Could you check a few things on this model? Use its own coordinates, in mm. A direction names the side the tool comes from. Round coordinates to 2 decimals unless told otherwise and drop trailing zeros. Loops run counter-clockwise (first coordinate to the right, second up) from the corner with the lowest first, then second, coordinate; pieces in that order, holes last.
from build123d import *

# Parameters (mm, degrees)
BASE_FLANGE1_DEPTH        = 3.175
EDGE_FLANGE1_DEPTH        = 95.421779032
EDGE_FLANGE1_BEND_DEPTH   = 168.275
EDGE_FLANGE1_BEND_2_DEPTH = 76.2


# Sheet-metal steps are written as plain solids
with BuildPart() as part:
    # Sketch1 → Base-Flange1 (new body)
    with BuildSketch(Plane(origin=(0, 0, 0), x_dir=(1, 0, 0), z_dir=(0, 1, 0))):
        Polygon((168.275, 79.375), (72.853220968, 79.375), (0, 28.362625496), (0, 6.35), (168.275, 6.35), align=None)
    extrude(amount=-BASE_FLANGE1_DEPTH)

    # Edge-Flange1 section (across the edge) → Edge-Flange1 (add)
    with BuildSketch(Plane(origin=(168.275, 0, -82.55), x_dir=(0, 0, 1), z_dir=(-1, 0, 0))):
        with BuildLine():
            Line((-3.175, 3.175), (-3.175, 15.875))
            Line((-3.175, 15.875), (0, 15.875))
            Line((0, 15.875), (0, 3.175))
            ThreePointArc((0, 3.175), (0.92993597, 0.92993597), (3.175, 0))
            Line((3.175, 0), (3.175, -3.175))
            ThreePointArc((3.175, -3.175), (-1.315128061, -1.315128061), (-3.175, 3.175))
        make_face()
    extrude(amount=EDGE_FLANGE1_DEPTH)

    # Edge-Flange1 section 2 (across the edge) → Edge-Flange1 bend (add)
    with BuildSketch(Plane(origin=(0, 0, -3.175), x_dir=(0, 0, -1), z_dir=(1, 0, 0))):
        with BuildLine():
            Line((-3.175, 3.175), (-3.175, 15.875))
            Line((-3.175, 15.875), (0, 15.875))
            Line((0, 15.875), (0, 3.175))
            ThreePointArc((0, 3.175), (0.92993597, 0.92993597), (3.175, 0))
            Line((3.175, 0), (3.175, -3.175))
            ThreePointArc((3.175, -3.175), (-1.315128061, -1.315128061), (-3.175, 3.175))
        make_face()
    extrude(amount=EDGE_FLANGE1_BEND_DEPTH)

    # Edge-Flange1 section 3 (across the edge) → Edge-Flange1 bend 2 (add)
    with BuildSketch(Plane(origin=(60.598280589, 0, -74.669957686), x_dir=(0.5735764363510473, 3.491481338843133e-15, 0.819152044288991), z_dir=(-0.819152044288991, 0, 0.5735764363510473))):
        with BuildLine():
            Line((-3.175, 3.175), (-3.175, 15.875))
            Line((-3.175, 15.875), (0, 15.875))
            Line((0, 15.875), (0, 3.175))
            ThreePointArc((0, 3.175), (0.92993597, 0.92993597), (3.175, 0))
            Line((3.175, 0), (3.175, -3.175))
            ThreePointArc((3.175, -3.175), (-1.315128061, -1.315128061), (-3.175, 3.175))
        make_face()
    extrude(amount=EDGE_FLANGE1_BEND_2_DEPTH)


solid = part.part
Item 1: If we section it at C-C, the plane z = -11: Please give me the cut outline in (x, y) (3 decimals), then the cut area to 3 significant figures.
Results list:
outline: (0, -3.175) - (168.275, -3.175) - (168.275, 0) - (0, 0) - close
area: 534 mm2
Item 2: If we section it at B-B, the plane x = 141.5: Please give me the cut outline in (y, z) (3 decimals), then the cut area to 3 significant figures.
Results list:
outline: (-3.175, -79.375) arc R6.35 ccw to (3.175, -85.725) - (15.875, -85.725) - (15.875, -82.55) - (3.175, -82.55) arc R3.175 cw to (0, -79.375) - (0, -6.35) arc R3.175 cw to (3.175, -3.175) - (15.875, -3.175) - (15.875, 0) - (3.175, 0) arc R6.35 ccw to (-3.175, -6.35) - close
area: 360 mm2
Item 3: If we section it at A-A, the plane y = 14: Please give me the cut outline in (x, z) (3 decimals).
Results list:
outline: (-3.642, -33.564) - (58.777, -77.271) - (60.598, -74.67) - (-1.821, -30.963) - close; (0, -3.175) - (168.275, -3.175) - (168.275, 0) - (0, 0) - close; (72.853, -85.725) - (168.275, -85.725) - (168.275, -82.55) - (72.853, -82.55) - close
Item 4: For faces 1 (the flat face through (121, 10, -82.55)), 2 (the cylindrical face through (30.3, 1, -52.4)), 3 (the flat face through (67.709, -1.565, -75.773)), 4 (the flat face through (0, -1, -10)), 5 (the flat face through (72.853, 6, -83)), which set-ups out of +Z, -Z, +X, -X, +Y, -Y let a thin tool reach every point of the face, with its end or its side?
Results list:
face 1: +X, -X, +Y
face 2: +X, +Y
face 3: -Z, +Y, -Y
face 4: +Z, -X, +Y, -Y
face 5: -Z, -X, +Y, -Y
Item 5: If I drill on line 1 along Z through (x, y) = (121, 6.5) (3 decimals); line 2 along Y through (x, z) = (100.5, -57) (3 decimals); line 3 along X through (y, z) = (0.75, -3.5) (3 decimals), over which ranges is the centre line in solid material (lowest first)?
Results list:
line 1: z = -85.725 to -82.55, -3.175 to 0
line 2: y = -3.175 to 0
line 3: x = 0 to 168.275
Item 6: If we section it at D-D, the plane x = 64: Please give me the cut outline in (y, z) (3 decimals).
Results list:
outline: (-3.175, -73.176) - (0, -73.176) - (0, -6.35) arc R3.175 cw to (3.175, -3.175) - (15.875, -3.175) - (15.875, 0) - (3.175, 0) arc R6.35 ccw to (-3.175, -6.35) - close
Item 7: Will these pins go through, and if not, where does the flat tip stop? pin 1 (5 mm diameter, centred on y = 2, z = -82.5, fed in from -X); pin 2 (10 mm diameter, centred on y = 12, z = -47, fed in from -X); pin 3 (4 mm diameter, centred on y = 14, z = -61, fed in from +X).
Results list:
pin 1: stops at x = 72.85
pin 2: stops at x = 8.41
pin 3: stops at x = 43.93
Item 8: We'd pull the mould along Z, two halves only. Please class faces 6 (the flat face through (83, 9, 0)), 7 (the cylindrical face through (29.1, -1.364, -54.159)), 8 (the flat face through (83, 10, -3.175)), 9 (the cylindrical face through (82.96, 0.955, -4.08)): released by +Z, released by -Z, zero draft, split by the parting line, or undercut.
Results list:
face 6: released by +Z
face 7: released by -Z
face 8: undercut
face 9: undercut
